Autodesk Inventor part; units mm, degrees
ref_plane "YZ Plane" through (0, 0, 0) normal (1, 0, 0) x (0, 1, 0)
ref_plane "XZ Plane" through (0, 0, 0) normal (0, 1, 0) x (-1, 0, 0)
ref_plane "XY Plane" through (0, 0, 0) normal (0, 0, 1) x (1, 0, 0)
sketch "Skizze1" plane through (0, 0, 0) normal (0, 0, 1) x (1, 0, 0)
  line L0 (10, 0) -> (-10, 0) construction
  line L1 (10, 8) -> (-10, 8)
  line L2 (-10, -8) -> (10, -8)
  arc A0 (10, -8) -> (10, 8) centre (10, 0) ccw
  arc A1 (-10, 8) -> (-10, -8) centre (-10, 0) ccw
  circle A2 centre (-10, 0) radius 1.75
  circle A3 centre (10, 0) radius 1.75
  point P0 (0, 0)
  dimension "d0" = 16
  dimension "d1" = 20
  dimension "d2" = 3.5
  dimension "d3" = 3.5
extrude "Extrusion1" add sketch "Skizze1" along normal blind 6
sketch "Skizze2" plane through (0, 0, 6) normal (0, 0, 1) x (1, 0, 0)
  line L0 (6, -6) -> (-6, -6)
  line L1 (-6, -6) -> (-6, 6)
  line L2 (-6, 6) -> (6, 6)
  line L3 (6, 6) -> (6, -6)
  line L4 (6, -6) -> (-6, 6) construction
  line L5 (-6, -6) -> (6, 6) construction
  point P0 (0, 0)
  dimension "d6" = 12
  dimension "d7" = 12
extrude "Extrusion2" cut sketch "Skizze2" against normal blind 4
sketch "Skizze3" plane through (-10, 8, 0) normal (0, 1, 0) x (1, 0, 0)
  line L0 (10, 1.2) -> (10, -7.2)
  line L1 (4, -6) -> (16, -6)
  line L2 (12.5, -4.5) -> (7.5, -4.5)
  line L3 (7.5, -4.5) -> (7.5, -6)
  line L4 (7.5, -6) -> (12.5, -6)
  line L5 (12.5, -6) -> (12.5, -4.5)
  line L6 (12.5, -4.5) -> (7.5, -6) construction
  line L7 (7.5, -4.5) -> (12.5, -6) construction
  point P0 (10, -5.25)
  dimension "d10" = 5
  dimension "d11" = 1.5
extrude "Extrusion3" cut sketch "Skizze3" against normal up to next
fillet "Rundung1" radius 0.5 2 edges at (-2.5, 7, 4.5) (2.5, 7, 4.5)
sketch "Skizze4" plane through (0, 0, 2) normal (0, 0, 1) x (1, 0, 0)
  line L0 (2.6, -6) -> (-2.6, -6)
  line L1 (-2.6, -6) -> (-2.6, 6)
  line L2 (-2.6, 6) -> (2.6, 6)
  line L3 (2.6, 6) -> (2.6, -6)
  line L4 (2.6, -6) -> (-2.6, 6) construction
  line L5 (-2.6, -6) -> (2.6, 6) construction
  line L6 (6, -6) -> (-6, -6)
  point P0 (0, 0)
  dimension "d15" = 5.2
extrude "Extrusion4" cut sketch "Skizze4" against normal blind 1
equation "\"d3\" = d2"
properties part number "LenkwinkelsensorAS5600"
Here's how the part is built. I have some questions about the finished solid (model axes, mm). A direction names the side the tool comes from. Round coordinates to 2 decimals unless told otherwise and drop trailing zeros. Loops run counter-clockwise (first coordinate to the right, second up) from the corner with the lowest first, then second, coordinate; pieces in that order, holes last. Notation, with made-up numbers: (14, 61) - (58, 61) arc R27 cw to (58, 88) - close; hole circle Ø2 at (55, -24). An arc over 180 degrees is marked (long way). One line per question, with ' | ' between items. Start each with the question number.
Q1. I want a section at B-B (y = 0). Write out the boundary of the cut face in (x, z), then the cut area to 3 significant figures.
Q2. Will these pins go through, and if not, where does the flat tip stop? pin 1 (1 mm diameter, centred on x = -3.5, y = -0.5, fed in from +Z); pin 2 (0.6 mm diameter, centred on x = -0.5, y = 7.5, fed in from +Z); pin 3 (1.5 mm diameter, centred on y = 4, z = 3, fed in from +X).
Q3. I want a section at A-A (z = 2.7). Write out the boundary of the cut face in (x, y), then the cut area to 3 significant figures.
Q4. For faces 5 (the flat face through (2.5, 7, 5.5)), 6 (the flat face through (6, 0, 4)), 7 (the cylindrical face through (-8.331, -0.526, 2.958)), which set-ups out of +Z, -Z, +X, -X, +Y, -Y let a thin tool reach every point of the face, with its end or its side?
Q5. I want a section at C-C (x = 9). Write out the boundary of the cut face in (y, z).
Q6. Please list where these lines run through material, in increasing order: line 1 (Y direction, x = 10, z = 4.65); line 2 (Y direction, x = 3.5, z = 5.7); line 3 (X direction, y = 0.25, z = 3.35). Write a range as [from, to].
Q7. We'd pull the mould along X, two halves only. Please class faces 1 (the cylindrical face through (-18, 0, 3)), 2 (the cylindrical face through (18, 0, 3)), 3 (the flat face through (-2.6, -0.1, 1.5)), 4 (the flat face through (0, -7, 6)): +X half, -X half, draft (parallel to the pull), parting line (faces both ways), or undercut.
Q8. I want a section at D-D (x = -4.5). Write out the boundary of the cut face in (y, z).
Response values:
1) outline: (-18, 0) - (-11.75, 0) - (-11.75, 6) - (-18, 6) - close; (-8.25, 0) - (8.25, 0) - (8.25, 6) - (6, 6) - (6, 2) - (2.6, 2) - (2.6, 1) - (-2.6, 1) - (-2.6, 2) - (-6, 2) - (-6, 6) - (-8.25, 6) - close; (11.75, 0) - (18, 0) - (18, 6) - (11.75, 6) - close | area: 121 mm²
2) pin 1: stops at z = 2 | pin 2: stops at z = 4.5 | pin 3: stops at x = 17.31
3) outline: (-10, -8) - (10, -8) arc R8 ccw to (10, 8) - (-10, 8) arc R8 ccw to start; hole circle Ø3.5 at (-10, 0); hole (-6, -6) - (6, -6) - (6, 6) - (-6, 6) - close; hole circle Ø3.5 at (10, 0) | area: 358 mm²
4) face 5: +Z, +Y | face 6: +Z | face 7: +Z, -Z
5) outline: (-8, 0) - (-1.44, 0) - (-1.44, 6) - (-8, 6) - close; (1.44, 0) - (8, 0) - (8, 6) - (1.44, 6) - close
6) line 1: y = [-8, -1.75], [1.75, 8] | line 2: y = [-8, -6], [6, 8] | line 3: x = [-18, -11.73], [-8.27, -6], [6, 8.27], [11.73, 18]
7) face 1: -X half | face 2: +X half | face 3: undercut | face 4: draft
8) outline: (-8, 0) - (8, 0) - (8, 6) - (6, 6) - (6, 2) - (-6, 2) - (-6, 6) - (-8, 6) - close
